Autodesk Inventor part; units mm, degrees
ref_plane "YZ Plane" through (0, 0, 0) normal (1, 0, 0) x (0, 1, 0)
ref_plane "XZ Plane" through (0, 0, 0) normal (0, 1, 0) x (-1, 0, 0)
ref_plane "XY Plane" through (0, 0, 0) normal (0, 0, 1) x (1, 0, 0)
sketch "Sketch1" plane through (0, 0, 0) normal (0, 0, 1) x (1, 0, 0)
  line L0 (-17.9772, -42.3695) -> (-21.9772, -42.3695) construction
  line L1 (-21.9772, -42.3695) -> (-21.9772, -36.3695) construction
  line L2 (-21.9772, -36.3695) -> (-17.9772, -36.3695) construction
  line L3 (-17.9772, -36.3695) -> (-17.9772, -42.3695) construction
  line L4 (52, -0.656) -> (44, -0.656) construction
  line L5 (44, -0.656) -> (44, 3.344) construction
  line L6 (44, 3.344) -> (52, 3.344) construction
  line L7 (52, 3.344) -> (52, -0.656) construction
  line L8 (-62, 48.621) -> (-62, 52.621) construction
  line L9 (-62, 52.621) -> (-54, 52.621) construction
  line L10 (-54, 52.621) -> (-54, 48.621) construction
  line L11 (-54, 48.621) -> (-62, 48.621) construction
  line L12 (-52, 7.344) -> (-52, 11.344) construction
  line L13 (-52, 11.344) -> (-44, 11.344) construction
  line L14 (-44, 11.344) -> (-44, 7.344) construction
  line L15 (-44, 7.344) -> (-52, 7.344) construction
  line L16 (62, 52.621) -> (62, 48.621) construction
  line L17 (62, 48.621) -> (54, 48.621) construction
  line L18 (54, 48.621) -> (54, 52.621) construction
  line L19 (54, 52.621) -> (62, 52.621) construction
  line L20 (44, 7.344) -> (44, 11.344) construction
  line L21 (44, 11.344) -> (52, 11.344) construction
  line L22 (52, 11.344) -> (52, 7.344) construction
  line L23 (52, 7.344) -> (44, 7.344) construction
  line L24 (-62, 56.621) -> (-62, 60.621) construction
  line L25 (-62, 60.621) -> (-54, 60.621) construction
  line L26 (-54, 60.621) -> (-54, 56.621) construction
  line L27 (-54, 56.621) -> (-62, 56.621) construction
  line L28 (-52, -0.656) -> (-52, 3.344) construction
  line L29 (-52, 3.344) -> (-44, 3.344) construction
  line L30 (-44, 3.344) -> (-44, -0.656) construction
  line L31 (-44, -0.656) -> (-52, -0.656) construction
  line L32 (62, 56.621) -> (54, 56.621) construction
  line L33 (54, 56.621) -> (54, 60.621) construction
  line L34 (54, 60.621) -> (62, 60.621) construction
  line L35 (62, 60.621) -> (62, 56.621) construction
  line L36 (95, 92.776) -> (95, 67.276) construction
  line L37 (-95, 92.776) -> (95, 92.776) construction
  line L38 (-95, 67.276) -> (-95, 92.776) construction
  spline S0 degree 4 poles (-93.2021, 32.276) (-94.3974, 41.3088) (-94.1998, 50.4639) (-95, 58.5765) (-95, 67.276) knots 0 0 0 0 0 1 1 1 1 1 construction
  spline S1 degree 3 poles (-93.2021, 32.276) (-92.477, 26.7964) (-92.3858, 18.3442) (-91.1679, 2.9086) (-90.2735, -4.0991) (-87.5297, -12.5723) (-86.3245, -15.3658) (-83.5784, -19.0417) (-82.333, -20.2665) (-79.6267, -21.887) (-78.3236, -22.3544) (-75.4283, -22.8138) (-73.9041, -22.7525) (-70.1581, -22.0875) (-67.9924, -21.2389) (-63.108, -18.9118) (-60.4378, -17.2966) (-54.8519, -14.6799) (-51.0186, -13.1408) (-44.4768, -12.6137) (-42.1843, -12.7653) (-38.5465, -13.8837) (-37.172, -14.5679) (-34.6876, -16.441) (-33.6448, -17.5823) (-32.7756, -18.8783) knots 0 0 0 0 1.658209 1.658209 2.939775 2.939775 3.538541 3.538541 3.905679 3.905679 4.202372 4.202372 4.52291 4.52291 5.00118 5.00118 5.654804 5.654804 6.203864 6.203864 6.490865 6.490865 6.688319 6.688319 6.886783 6.886783 6.886783 6.886783 construction
  spline S2 degree 4 poles (95, 67.276) (95, 55.7504) (92.5859, 37.7114) (100.8312, 0.406) (16.3507, -5.0368) (37.7982, -57.0134) (0, -92.776) (-31.6805, -62.8016) (-26.5791, -34.2881) (-31.0379, -21.8211) (-32.7756, -18.8783) knots 0 0 0 0 0 0.141322 0.242902 0.345989 0.449799 0.550201 0.654011 0.69056 0.69056 0.69056 0.69056 0.69056 construction
  line L39 (-40, 82.776) -> (-44, 82.776) construction
  line L40 (-40, 62.776) -> (-40, 82.776) construction
  line L41 (-44, 62.776) -> (-40, 62.776) construction
  line L42 (-44, 82.776) -> (-44, 62.776) construction
  line L43 (-40, 22.776) -> (-40, 42.776) construction
  line L44 (-44, 22.776) -> (-40, 22.776) construction
  line L45 (-44, 42.776) -> (-44, 22.776) construction
  line L46 (-40, 42.776) -> (-44, 42.776) construction
  line L47 (-10, 12.776) -> (-30, 12.776) construction
  line L48 (-10, 8.776) -> (-10, 12.776) construction
  line L49 (-30, 8.776) -> (-10, 8.776) construction
  line L50 (-30, 12.776) -> (-30, 8.776) construction
  line L51 (44, 82.776) -> (40, 82.776) construction
  line L52 (44, 62.776) -> (44, 82.776) construction
  line L53 (40, 62.776) -> (44, 62.776) construction
  line L54 (40, 82.776) -> (40, 62.776) construction
  line L55 (44, 22.776) -> (44, 42.776) construction
  line L56 (40, 22.776) -> (44, 22.776) construction
  line L57 (40, 42.776) -> (40, 22.776) construction
  line L58 (44, 42.776) -> (40, 42.776) construction
  line L59 (30, 12.776) -> (10, 12.776) construction
  line L60 (30, 8.776) -> (30, 12.776) construction
  line L61 (10, 8.776) -> (30, 8.776) construction
  line L62 (10, 12.776) -> (10, 8.776) construction
  circle A0 centre (-78.75, 27.8364) radius 1.5 construction
  circle A1 centre (-58.125, 15.9285) radius 1.5 construction
  circle A2 centre (-71.875, 15.9285) radius 1.5 construction
  circle A3 centre (-71.875, 39.7442) radius 1.5 construction
  circle A4 centre (-58.125, 39.7442) radius 1.5 construction
  circle A5 centre (-51.25, 27.8364) radius 1.5 construction
  circle A6 centre (-65, 27.8364) radius 10.5 construction
  circle A7 centre (-8.625, -30.663) radius 1.5 construction
  circle A8 centre (8.625, -30.663) radius 1.5 construction
  circle A9 centre (17.25, -15.724) radius 1.5 construction
  circle A10 centre (8.625, -0.7851) radius 1.5 construction
  circle A11 centre (-8.625, -0.7851) radius 1.5 construction
  circle A12 centre (-17.25, -15.724) radius 1.5 construction
  circle A13 centre (6.875, -45.3162) radius 1.5 construction
  circle A14 centre (13.75, -57.224) radius 1.5 construction
  circle A15 centre (0, -57.224) radius 10.5 construction
  circle A16 centre (-6.875, -69.1319) radius 1.5 construction
  circle A17 centre (6.875, -69.1319) radius 1.5 construction
  circle A18 centre (-6.875, -45.3162) radius 1.5 construction
  circle A19 centre (-13.75, -57.224) radius 1.5 construction
  circle A20 centre (58.125, 15.9285) radius 1.5 construction
  circle A21 centre (71.875, 15.9285) radius 1.5 construction
  circle A22 centre (78.75, 27.8364) radius 1.5 construction
  circle A23 centre (71.875, 39.7442) radius 1.5 construction
  circle A24 centre (58.125, 39.7442) radius 1.5 construction
  circle A25 centre (51.25, 27.8364) radius 1.5 construction
  circle A26 centre (0, -15.724) radius 14 construction
  circle A27 centre (65, 27.8364) radius 10.5 construction
  circle A28 centre (8.9, 77.626) radius 1.175
  circle A29 centre (8.9, 68.126) radius 1.175
  line L63 (6, 62.976) -> (15.4, 62.976)
  line L64 (15.4, 62.976) -> (15.4, 82.776)
  line L65 (15.4, 82.776) -> (6, 82.776)
  line L66 (6, 82.776) -> (6, 62.976)
  point P0 (0, 0)
  dimension "d0" = 24.6
  dimension "d1" = 2.35
  dimension "d2" = 9.5
  dimension "d3" = 19.8
  dimension "d4" = 9.4
  dimension "d5" = 5.15
  dimension "d6" = 2.9
  dimension "d7" = 10
extrude "Extrusion1" add sketch "Sketch1" along normal blind 4
fillet "Fillet1" radius 2 4 edges at (6, 62.976, 2) (15.4, 62.976, 2) (15.4, 82.776, 2) (6, 82.776, 2)
properties part number "Door_LimitSwitch_Offset" material "MDF Medium Density Fiberboard"
Model file for the job. Use its own axes, mm. Coordinates: 2 decimals unless noted, no trailing zeros. Write each loop counter-clockwise with the first axis right and the second up, starting at its lowest first coordinate (ties: lowest second). Pieces come first, ordered by that corner, then holes. Notation, with made-up numbers: (11, -37.5) - (16, -37.5) arc R18 ccw to (16, -19.5) - close; hole circle Ø6 at (-37, 34.5). An arc over 180 degrees is marked (long way). Write each question's results on one line, items separated by ' | '. Start each with the question number.
1) Cut at C-C (x = 14.25). Write the cut outline in (y, z), then the cut area to 3 significant figures.
2) Mould opens along Y. For faces 1 (the face through (15.4, 73, 2)), 2 (the face through (8.645, 78.773, 1.972)), 3 (the face through (6.601, 82.206, 2.028)) say: pulls with the +Y half, pulls with the -Y half, needs draft (parallel to the pull), parting line crosses it, or undercut.
3) Probe line 1 along Y through (x, z) = (8.9, 0.8); line 2 along Y through (x, z) = (8.5, 1.9); line 3 along X through (y, z) = (67.5, 1.65). List the from-to ranges inside material, lowest first. Write a range as from..to.
4) Cut at B-B (z = 2.9). Write the cut outline in (x, y) (3 decimals).
5) Cut at A-A (x = 8.9). Write the cut outline in (y, z).
6) Flat gauge pin, fed straight in: P1, Ø2, axis at x = 8.9, y = 77.626, coming from the -Z side. Where does the tip first touch, or does it go through?
Returned:
1) outline: (63.17, 0) - (82.59, 0) - (82.59, 4) - (63.17, 4) - close | area: 77.7 mm^2
2) face 1: needs draft | face 2: undercut | face 3: pulls with the +Y half
3) line 1: 62.98..66.95, 69.3..76.45, 78.8..82.78 | line 2: 62.98..67.02, 69.23..76.52, 78.73..82.78 | line 3: 6..7.91, 9.89..15.4
4) outline: (6, 64.976) arc R2 ccw to (8, 62.976) - (13.4, 62.976) arc R2 ccw to (15.4, 64.976) - (15.4, 80.776) arc R2 ccw to (13.4, 82.776) - (8, 82.776) arc R2 ccw to (6, 80.776) - close; hole circle Ø2.35 at (8.9, 68.126); hole circle Ø2.35 at (8.9, 77.626)
5) outline: (62.98, 0) - (66.95, 0) - (66.95, 4) - (62.98, 4) - close; (69.3, 0) - (76.45, 0) - (76.45, 4) - (69.3, 4) - close; (78.8, 0) - (82.78, 0) - (82.78, 4) - (78.8, 4) - close
6) P1: through
